Geometry check sheet. Reference: the model listing, model coordinates, mm. A direction names the side the tool comes from. Coordinates: 2 decimals unless noted, no trailing zeros. Write each loop counter-clockwise with the first axis right and the second up, starting at its lowest first coordinate (ties: lowest second). Pieces come first, ordered by that corner, then holes. Notation, with made-up numbers: M 66,-29 L 89,-29 A15 ccw 89,0 Z; hole C -30.75,36 d6. An arc over 180 degrees is marked long. Write item = value, one per line. Start each with the question number.
Autodesk Inventor part; units mm, degrees
ref_plane "YZ Plane" through (0, 0, 0) normal (1, 0, 0) x (0, 1, 0)
ref_plane "XZ Plane" through (0, 0, 0) normal (0, 1, 0) x (-1, 0, 0)
ref_plane "XY Plane" through (0, 0, 0) normal (0, 0, 1) x (1, 0, 0)
sketch "Sketch1" plane through (0, 0, 0) normal (0, 0, 1) x (1, 0, 0)
  line L0 (-110, 70) -> (110, 70) construction
  line L1 (110, 70) -> (110, -70) construction
  line L2 (110, -70) -> (-110, -70) construction
  line L3 (-110, -70) -> (-110, 70) construction
  circle A0 centre (-90, 55) radius 5
  circle A1 centre (-90, -55) radius 5
  circle A2 centre (90, -55) radius 5
  circle A3 centre (-10, 45) radius 5
  line L4 (-67, 0) -> (-42, 0) construction
  line L5 (-42, 0) -> (-42, -30) construction
  line L6 (-42, -30) -> (-67, -30) construction
  line L7 (-67, -30) -> (-67, 0) construction
  circle A4 centre (-54.5, -19) radius 10 construction
  arc A5 (-76.2883, 61.082) -> (-104.3936, 50.7781) centre (-90, 55) ccw
  arc A6 (-99.9402, -53.9078) -> (-88.1099, -64.8197) centre (-90, -55) ccw
  arc A7 (-100, -55) -> (-105, 55) centre (-644.4063, -24.6321) ccw
  line L8 (-34.9568, 51.6958) -> (-68.1552, 21.4315)
  line L9 (-75.2957, 53.6513) -> (-76.519, 25.3424)
  line L10 (-78.8103, -29) -> (-79.758, -49.8907)
  arc A8 (80, -54.9687) -> (97.6304, -48.5365) centre (90, -55) ccw
  line L11 (5.2335, 60.5405) -> (97.6304, -48.5365)
  arc A9 (5.2335, 60.5405) -> (-24.6607, 61.082) centre (-10, 45) ccw
  arc A10 (-76.519, 25.3424) -> (-68.1552, 21.4315) centre (-71.5236, 25.1265) ccw
  line L12 (-76.2883, 61.082) -> (-24.6607, 61.082)
  line L13 (-72.7981, 56.0433) -> (-36.641, 56.0433)
  arc A11 (-72.7981, 56.0433) -> (-75.2957, 53.6513) centre (-72.7981, 53.5433) ccw
  arc A12 (-34.9568, 51.6958) -> (-36.641, 56.0433) centre (-36.641, 53.5433) ccw
  arc A13 (90, -65) -> (-90.7731, -64.9701) centre (-0.647, -1637.996) ccw
  arc A14 (-20.0638, 28.3489) -> (-21.4839, -47.6911) centre (99.5478, -11.9183) ccw
  arc A15 (-0.4705, -47.7594) -> (-0.8289, 17.7317) centre (-195.1328, -16.0782) ccw
  circle A16 centre (-63.5274, -9.3914) radius 3 construction
  circle A17 centre (-57.919, -6.3914) radius 3 construction
  circle A18 centre (-51.0643, -6.3914) radius 3 construction
  circle A19 centre (-45.5038, -9.3914) radius 3 construction
  arc A20 (-23.0905, 31.5585) -> (-78.8103, -29) centre (-2.7481, -43.0717) ccw
  line L14 (-77.2605, -52.504) -> (-25.0801, -52.504)
  line L15 (3.2308, -52.1118) -> (58.9703, -52.1118)
  arc A21 (-20.0638, 28.3489) -> (-23.0905, 31.5585) centre (-22.4331, 29.1465) ccw
  arc A22 (3.7556, 19.4828) -> (-0.8289, 17.7317) centre (1.6341, 18.1603) ccw
  arc A23 (-0.4705, -47.7594) -> (3.2308, -52.1118) centre (3.2308, -48.3618) ccw
  arc A24 (-25.0801, -52.504) -> (-21.4839, -47.6911) centre (-25.0801, -48.754) ccw
  arc A25 (58.9703, -52.1118) -> (61.9167, -43.0722) centre (58.9703, -47.1118) ccw
  arc A26 (3.7556, 19.4828) -> (61.9167, -43.0722) centre (194.066, 138.1102) ccw
  arc A27 (75.297, -52.1118) -> (80, -54.9687) centre (194.066, 138.1102) ccw
  arc A28 (-79.758, -49.8907) -> (-77.2605, -52.504) centre (-77.2605, -50.004) ccw
  point P0 (0, 0)
  dimension "d1" = 70
  dimension "d2" = 70
  dimension "d3" = 110
  dimension "d4" = 110
  dimension "d5" = 10
  dimension "d6" = 10
  dimension "d7" = 10
  dimension "d8" = 10
  dimension "d9" = 55
  dimension "d10" = 55
  dimension "d11" = 55
  dimension "d12" = 180
  dimension "d13" = 90
  dimension "d15" = 10
  dimension "d16" = 45
  dimension "d17" = 42
  dimension "d18" = 30
  dimension "d19" = 0
  dimension "d20" = 25
  dimension "d21" = 20
  dimension "d25" = 19
  dimension "d26" = 12.5
  dimension "d67" = 90
  dimension "d68" = 30
  dimension "d70" = 20
  dimension "d71" = 20
  dimension "d74" = 10
  dimension "d75" = 5
  dimension "d76" = 5
  dimension "d77" = 6
  dimension "d78" = 6
  dimension "d79" = 6
  dimension "d80" = 6
  dimension "d81" = 5
  dimension "d82" = 5
  dimension "d83" = 7.5
  dimension "d84" = 7.5
  dimension "d85" = 10
  dimension "d88" = 5
extrude "Extrusion8" add sketch "Sketch1" along normal blind 9.4 contours L12 A9 L11 A8 A13 A6 A7 A5
equation "\"d26\" = 0.5 * d20"
properties part number "Bracket Concept MK10"
Q1. Set-up check for faces 1 (the face through (-51, 61.082, 5)), 2 (the face through (30.24, -15.03, 4.63)), 3 (the face through (99.14, -59.06, 4.63)): record each of +Z, -Z, +X, -X, +Y, -Y from which the full face is reachable in a straight line by a thin tool's end or side.
Q2. Cross-section at B-B on x = -10. Enter the section's corners in (y, z).
Q3. Draft check along X on faces 4 (the face through (0.404, -50.826, 4.634)), 5 (the face through (-4, -12, 0)), 6 (the face through (-60.081, 8.855, 4.634)), 7 (the face through (-97.268, -61.869, 4.634)). Enter one of: pulls with the +X half, pulls with the -X half, needs draft (parallel to the pull), parting line crosses it, or undercut.
Q4. Cross-section at C-C on z = 2.5. Count the separate pieces of the cut face and the enclosed holes in it, and give its area (3 significant figures).
Q5. Scan lines: L1, parallel to Y at x = -90, z = 6; L2, parallel to Y at x = -10, z = 5; L3, parallel to Y at x = -86, z = 7.25. Record each from-to range of solid material in increasing order.
Q6. Cross-section at D-D on x = -44. Enter the section's corners in (y, z), and give its area (3 significant figures).
Q7. Gauge pin test, flat ends, axial feed: pin 1 (4.5 mm diameter, centred on x = -51, z = 4, fed in from +Y); pin 2 (4 mm diameter, centred on x = -12.5, z = 3.5, fed in from -Y); pin 3 (4 mm diameter, centred on x = 54.5, z = 4, fed in from -Y). Record the tip position at first contact, or that the pin passes through.
Q8. Cross-section at A-A on y = 45. Enter the section's corners in (x, z), and give its area (3 significant figures).
Values found:
q1.face_1 = +Z, -Z, +Y
q1.face_2 = +Z, -Z
q1.face_3 = +Z, -Z, +X
q2.outline = M -62.42,0 L 40,0 L 40,9.4 L -62.42,9.4 Z; M 50,0 L 66.76,0 L 66.76,9.4 L 50,9.4 Z
q3.face_4 = undercut
q3.face_5 = needs draft
q3.face_6 = undercut
q3.face_7 = pulls with the -X half
q4.separate_pieces = 1
q4.enclosed_holes = 7
q4.area = 12,800 mm²
q5.L1 = -64.93 to -60, -50 to 50, 60 to 70
q5.L2 = -62.42 to 40, 50 to 66.76
q5.L3 = -64.7 to -58, -52 to 52, 58 to 69.46
q6.outline = M -62.99,0 L -52.5,0 L -52.5,9.4 L -62.99,9.4 Z; M 22.36,0 L 43.45,0 L 43.45,9.4 L 22.36,9.4 Z; M 56.04,0 L 61.08,0 L 61.08,9.4 L 56.04,9.4 Z
q6.area = 344 mm²
q7.pin_1 = 61.08
q7.pin_2 = -62.45
q7.pin_3 = -63.43
q8.outline = M -103.62,0 L -75.67,0 L -75.67,9.4 L -103.62,9.4 Z; M -42.3,0 L -15,0 L -15,9.4 L -42.3,9.4 Z; M -5,0 L 18.4,0 L 18.4,9.4 L -5,9.4 Z
q8.area = 739 mm²
